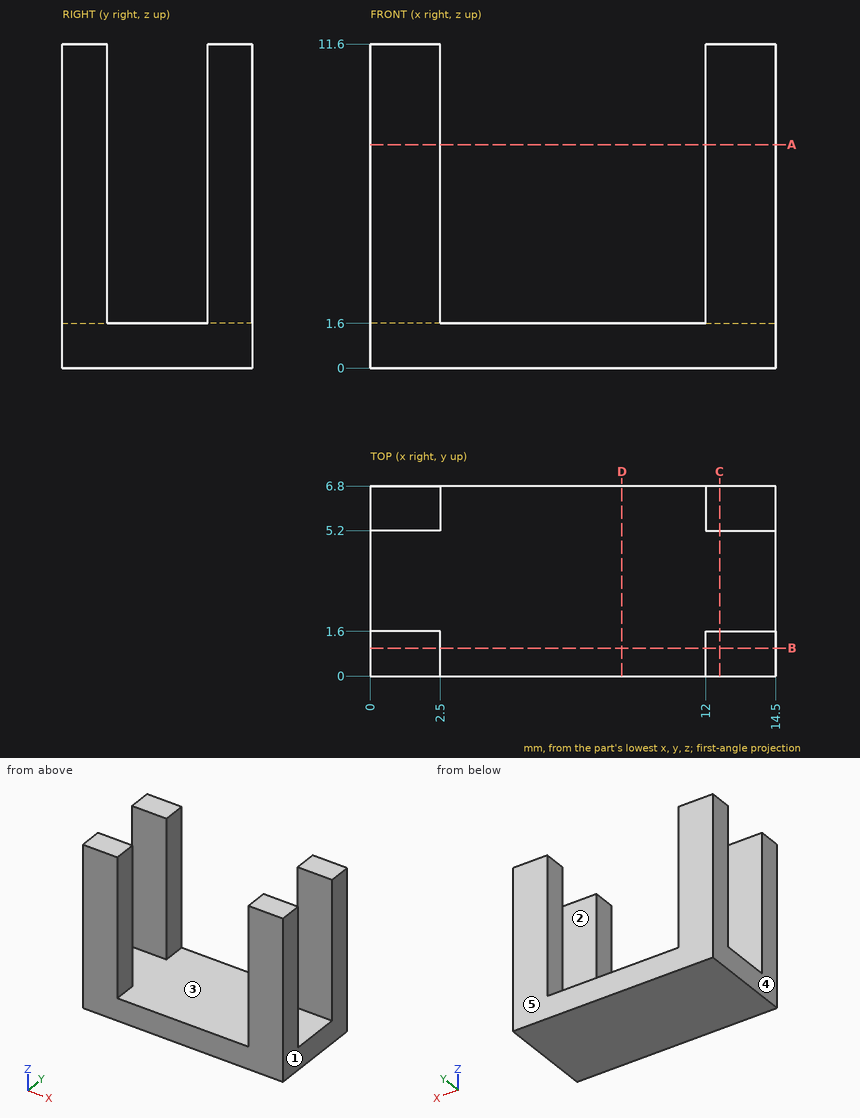
Print and shaded views of the part. All mm, measured from the part's lowest x, y and z. A direction names the side the tool comes from. Round coordinates to 2 decimals unless told otherwise and drop trailing zeros. Write each loop counter-clockwise with the first axis right and the second up, starting at its lowest first coordinate (ties: lowest second). Pieces come first, ordered by that corner, then holes. Notation, with made-up numbers: M 79,31.5 L 115,31.5 A31 cw 115,55.5 Z; hole C -38,30 d2. An arc over 180 degrees is marked long. Use a Markdown table: item, result. Add a question column.
1. Drill centre lines: probe 1 along Z at (x, y) = (7.25, 5); probe 2 along X at (y, z) = (6, 7.25). Where is each one in solid material? Low to high.
2. Pull direction X, two halves, no side cores. Call the marked faces 3, 4 and 5: released by +X, released by -X, zero draft, split by the parting line, or undercut.
3. Slice it at D-D on x = 9. Give the cut face in (y, z).
4. Slice it at B-B on y = 1. Give the cut face in (x, z).
5. Flat gauge pins, fed straight in: P1, Ø3.5, axis at x = 4.5, y = 4, coming from the +Z side; P2, Ø1.3, axis at y = 1, z = 6.5, coming from the -X side. Where does each tip first touch, or does it go through?
6. 3-axis set-ups, long thin cutter, end or side, ignore diameter. For the marked faces 1 and 2: which of +Z, -Z, +X, -X, +Y, -Y reach the whole face in a straight line?
7. Slice it at C-C on x = 12.5. Give the cut face in (y, z).
8. Slice it at A-A on z = 8. Give the cut face in (x, y).
Reply:
| question | item | result |
|---|---|---|
| 1 | probe 1 | z = 0 to 1.6 |
| 1 | probe 2 | x = 0 to 2.5, 12 to 14.5 |
| 2 | face 3 | undercut |
| 2 | face 4 | released by -X |
| 2 | face 5 | zero draft |
| 3 | outline | M 0,0 L 6.8,0 L 6.8,1.6 L 0,1.6 Z |
| 4 | outline | M 0,0 L 14.5,0 L 14.5,11.6 L 12,11.6 L 12,1.6 L 2.5,1.6 L 2.5,11.6 L 0,11.6 Z |
| 5 | P1 | stops at z = 1.6 |
| 5 | P2 | stops at x = 0 |
| 6 | face 1 | +Z, -Z, +X, +Y, -Y |
| 6 | face 2 | +Z, +X, -X |
| 7 | outline | M 0,0 L 6.8,0 L 6.8,11.6 L 5.2,11.6 L 5.2,1.6 L 1.6,1.6 L 1.6,11.6 L 0,11.6 Z |
| 8 | outline | M 0,0 L 2.5,0 L 2.5,1.6 L 0,1.6 Z; M 0,5.2 L 2.5,5.2 L 2.5,6.8 L 0,6.8 Z; M 12,0 L 14.5,0 L 14.5,1.6 L 12,1.6 Z; M 12,5.2 L 14.5,5.2 L 14.5,6.8 L 12,6.8 Z |
